Autodesk Inventor part; units mm, degrees
ref_plane "YZ Plane" through (0, 0, 0) normal (1, 0, 0) x (0, 1, 0)
ref_plane "XZ Plane" through (0, 0, 0) normal (0, 1, 0) x (-1, 0, 0)
ref_plane "XY Plane" through (0, 0, 0) normal (0, 0, 1) x (1, 0, 0)
sketch "スケッチ1" plane through (0, 0, 0) normal (1, 0, 0) x (0, 1, 0)
  line L0 (7, 5.6) -> (0, 5.6)
  line L1 (0, 5.6) -> (0, -5.6)
  line L2 (0, -5.6) -> (7, -5.6)
  line L3 (7, -5.6) -> (7, 5.6)
  line L4 (7, 5.6) -> (-6, 5.6)
  line L5 (-6, 5.6) -> (-6, 13.6)
  line L6 (-6, 13.6) -> (7, 13.6)
  line L7 (7, 13.6) -> (7, 5.6)
  line L8 (7, -5.6) -> (-6, -5.6)
  line L9 (-6, -5.6) -> (-6, -13.6)
  line L10 (-6, -13.6) -> (7, -13.6)
  line L11 (7, -13.6) -> (7, -5.6)
  arc A0 (0, 3.5) -> (0, 5.6) centre (0, 4.55) ccw
  arc A1 (0, -5.6) -> (0, -3.5) centre (0, -4.55) ccw
  point P0 (0, 0)
  point P1 (0, 0)
  point P2 (0, 5.6)
  point P3 (0, 5.6)
  dimension "d0" = 7
  dimension "d1" = 11.2
  dimension "d2" = 13
  dimension "d3" = 13
  dimension "d4" = 8
  dimension "d5" = 8
  dimension "d8" = 1.05
extrude "押し出し1" add sketch "スケッチ1" along normal blind 5 contours L3 L2 A1 L1 A0 L0 | L0 L4 L5 L6 L7 | L11 L10 L9 L8 L2
sketch "スケッチ2" plane through (0, 7, 13.6) normal (0, 1, 0) x (1, 0, 0)
  line L0 (0, 27.2) -> (0, 0)
  line L1 (0, 0) -> (5, 0)
  line L2 (5, 27.2) -> (5, 0)
  line L3 (0, 27.2) -> (5, 27.2)
  line L4 (2.5, 0) -> (2.5, 27.2) construction
  circle A0 centre (2.5, 3) radius 1.25
  circle A1 centre (2.5, 24.2) radius 1.25
  point P0 (0, 13.6)
  dimension "d9" = 2.5
  dimension "d10" = 2.5
  dimension "d11" = 3
  dimension "d12" = 3
extrude "押し出し2" cut sketch "スケッチ2" against normal up to surface (13 mm away) contours A0 | A1
sketch "スケッチ3" plane through (0, -6, 13.6) normal (0, 0, 1) x (1, 0, 0)
  circle A0 centre (2.5, 3) radius 1.5
  line L0 (0, 0) -> (5, 0)
  point P0 (0, 6)
  point P1 (2.5, 0)
  dimension "d15" = 3
  dimension "d16" = 3
extrude "押し出し3" cut sketch "スケッチ3" against normal up to surface (27.2 mm away)
fillet "フィレット1" radius 1 4 edges at (2.5, -6, -5.6) (2.5, -6, -13.6) (2.5, -6, 5.6) (2.5, -6, 13.6)
equation "\"d3\" = d2"
equation "\"d5\" = d4"
equation "\"d10\" = d9"
equation "\"d12\" = d11"
properties part number "ウィング土台" material "アルミニウム 2014-T4"
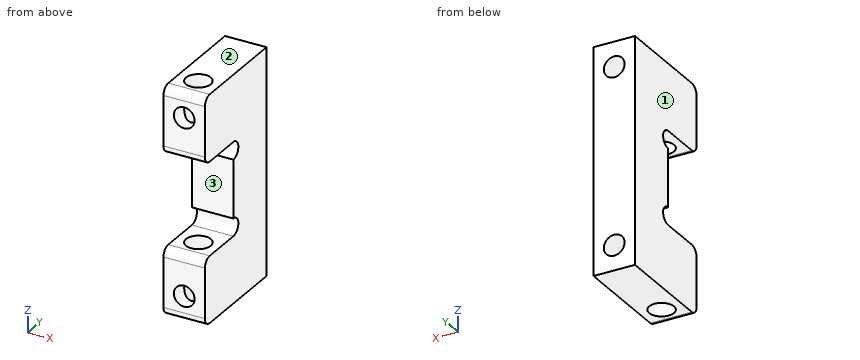
Source: CAD feature listing. Evaluate the final solid. Frame: model axes, mm. Face numbers are marked on the shaded views. Round coordinates to 2 decimals unless told otherwise and drop trailing zeros. Loops run counter-clockwise (first coordinate to the right, second up) from the corner with the lowest first, then second, coordinate; pieces in that order, holes last. Notation, with made-up numbers: M 78,72.5 L 96,72.5 A25 cw 96,107.5 Z; hole C 48,-19.75 d5. An arc over 180 degrees is marked long. Use a Markdown table: item, result. Add a question column.
1. Section query C-C on x = 4.25. Return the cut outline in (y, z).
2. Section query A-A on y = 0.25. Return the cut outline in (x, z), then the cut area to 3 significant figures.
3. Section query D-D on z = -2.25. Return the cut outline in (x, y).
4. Contact query for flat-ended pins moving along their axis: P1, Ø2.5, axis at x = 1.5, z = -1.5, coming from the -Y side; P2, Ø2, axis at x = 2.5, z = 10.6, coming from the -Y side. Output: stop coordinate, or through.
5. Line query: line 1 (Z direction, x = 2.5, y = 3.75); line 2 (X direction, y = 1.5, z = 10.6); line 3 (Z direction, x = 0.5, y = -1.5). Output: solid intervals per line, ascending.
6. Mould query, pull axis Z, two halves, no side actions, for the marked faces 1, 2 and 3. Classes: pulls with the +Z half, pulls with the -Z half, needs draft (parallel to the pull), parting line crosses it, or undercut.
7. Section query B-B on y = 3. Return the cut outline in (x, z).
Reported:
| question | item | result |
|---|---|---|
| 1 | outline | M -6,-12.6 A1 ccw -5,-13.6 L 7,-13.6 L 7,13.6 L -5,13.6 A1 ccw -6,12.6 L -6,6.6 A1 ccw -5,5.6 L 0,5.6 A1.05 cw 0,3.5 L 0,-3.5 A1.05 cw 0,-5.6 L -5,-5.6 A1 ccw -6,-6.6 Z |
| 2 | outline | M 0,-13.6 L 5,-13.6 L 5,-5.57 L 0,-5.57 Z; M 0,-3.53 L 5,-3.53 L 5,3.53 L 0,3.53 Z; M 0,5.57 L 5,5.57 L 5,13.6 L 0,13.6 Z; hole C 2.5,-10.6 d2.5; hole C 2.5,10.6 d2.5 |
| 2 | area | 106 mm² |
| 3 | outline | M 0,0 L 5,0 L 5,7 L 0,7 Z |
| 4 | P1 | stops at y = 0 |
| 4 | P2 | passes through |
| 5 | line 1 | z = -13.6 to -11.85, -9.35 to 9.35, 11.85 to 13.6 |
| 5 | line 2 | x = 0 to 1.25, 3.75 to 5 |
| 5 | line 3 | z = -13.6 to -5.6, 5.6 to 13.6 |
| 6 | face 1 | needs draft |
| 6 | face 2 | pulls with the +Z half |
| 6 | face 3 | undercut |
| 7 | outline | M 0,-13.6 L 5,-13.6 L 5,13.6 L 0,13.6 Z; hole C 2.5,-10.6 d2.5; hole C 2.5,10.6 d2.5 |
